The model under review builds one solid part; all positions refer to its coordinate system, in mm. Give positions to 0.01 mm unless a question says otherwise; leave off trailing zeros. Order: outer loops, then holes, each group sorted by start corner. A loop starts at its lowest first (then second) coordinate and runs counter-clockwise, first axis right, second up.
```python
from build123d import *

# Parameters (mm, degrees)
SKETCH1_W                                = 200
SKETCH1_H                                = 40
RECTANGULAR_BAR_40_W_X_200_L_X_15D_DEPTH = 15
NOTCH_CUT_OUT_DEPTH                      = 15


with BuildPart() as part:
    # Sketch1 → Rectangular Bar (40 W x 200 L x 15D) (new body)
    with BuildSketch(Plane.XY):
        Rectangle(SKETCH1_W, SKETCH1_H)
    extrude(amount=RECTANGULAR_BAR_40_W_X_200_L_X_15D_DEPTH)

    # Notch → Notch cut out (cut)
    with BuildSketch(Plane.XY.offset(15)):
        with BuildLine():
            Line((2, 20), (2, 12))
            ThreePointArc((2, 12), (0, 10), (-2, 12))
            Line((-2, 12), (-2, 20))
            Line((-2, 20), (2, 20))
        make_face()
        with BuildLine():
            Line((-2, -20), (-2, -12))
            ThreePointArc((-2, -12), (0, -10), (2, -12))
            Line((2, -12), (2, -20))
            Line((2, -20), (-2, -20))
        make_face()
    extrude(amount=-NOTCH_CUT_OUT_DEPTH, mode=Mode.SUBTRACT)


solid = part.part
```
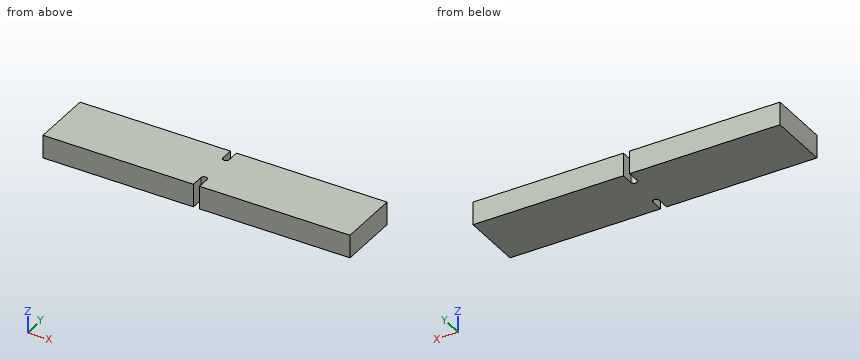
Item 1: For line 1 (X direction, y = 15, z = 12); line 2 (X direction, y = 10.5, z = 14), list the stretches that pass through material, from the lowest coordinate up.
Values found:
line 1: x = -100 to -2, 2 to 100
line 2: x = -100 to -1.32, 1.32 to 100
Item 2: Take a section at B-B (x = 0). Give the boundary of the cut face in (y, z).
Values found:
outline: (-10, 0) - (10, 0) - (10, 15) - (-10, 15) - close
Item 3: Take a section at A-A (y = 15). Give the boundary of the cut face in (x, z), and give its area (3 significant figures).
Values found:
outline: (-100, 0) - (-2, 0) - (-2, 15) - (-100, 15) - close; (2, 0) - (100, 0) - (100, 15) - (2, 15) - close
area: 2,940 mm2
